The listing builds one solid part. Answer for the finished solid, in the listing's coordinates (mm). A direction names the side the tool comes from. Give positions to 0.01 mm unless a question says otherwise; leave off trailing zeros. Write each loop counter-clockwise with the first axis right and the second up, starting at its lowest first coordinate (ties: lowest second). Pieces come first, ordered by that corner, then holes. Notation, with made-up numbers: (6.25, 86.25) - (18.25, 86.25) arc R6 ccw to (18.25, 90.25) - close; hole circle Ø7 at (-28.5, 45). An arc over 180 degrees is marked (long way). Write each question's results on one line, items separated by ' | '. Start each with the question number.
Q1. Section B-B (y = 0) is taken. Determine the outline of the cut face in (x, z), plus the area to 4 significant figures.
Q2. For faces 1 (the face through (-7.215, -5.599, 6.084)), 2 (the face through (6, 6.5, 6.7)), 3 (the face through (-6, 6.5, 6.7)), determine the directions among +Z, -Z, +X, -X, +Y, -Y from which every point of the face is accessible in a straight line to the end or side of a thin tool.
Q3. Section C-C (z = 6) is taken. Determine the outline of the cut face in (x, y).
Q4. Section D-D (y = 6) is taken. Determine the outline of the cut face in (x, z), plus the area to 3 significant figures.
Q5. Flat-ended cylindrical pins translate along their axes: pin 1 Ø4 at (y, z) = (13, 5.5) entering from +X; pin 2 Ø5 at (x, z) = (4.5, 7) entering from +Y; pin 3 Ø2 at (x, y) = (-2, 9.5) entering from +Z. Find the tip coordinate at first contact, or state that the pin passes through.
Q6. Find the intervals of material crossed by probe 1 along Y at (x, z) = (0, 2.5); probe 2 along Z at (x, y) = (-4.9, 0); probe 3 along Z at (x, y) = (1.25, 9.25), in increasing order.
Q7. For a pull along Y with two mould halves and no side action, classify faces 4 (the face through (2, 4, 12)), 5 (the face through (3.926, 1.628, 5.916)), 6 (the face through (0, 8, 7)) as pulls with the +Y half, pulls with the -Y half, needs draft (parallel to the pull), parting line crosses it, or undercut.
Q8. Section A-A (x = 0) is taken. Determine the outline of the cut face in (y, z), plus the area to 3 significant figures.
Autodesk Fusion 360 part; units mm, degrees
sketch "スケッチ1" plane through (0, 0, 0) normal (0, 0, 1) x (1, 0, 0)
  line L0 (7.5, 16) -> (-7.5, 16)
  line L1 (-7.5, 16) -> (-7.5, -5.9)
  line L2 (-7.5, -5.9) -> (7.5, -5.9)
  line L3 (7.5, -5.9) -> (7.5, 16)
  line L4 (7.5, 16) -> (-7.5, -5.9) construction
  line L5 (-7.5, 16) -> (7.5, -5.9) construction
  circle A0 centre (0, 0) radius 4.25
  line L6 (-7.5, 5) -> (-4.5, 8)
  line L7 (-4.5, 8) -> (4.5, 8)
  line L8 (4.5, 8) -> (7.5, 5)
  point P0 (0, 5.05)
  dimension "d1" = 15
  dimension "d2" = 21.9
  dimension "d3" = 8.5
  dimension "d4" = 5.9
  dimension "d5" = 13.9
  dimension "d6" = 45
  dimension "d7" = 45
  dimension "d8" = 3
  dimension "d9" = 3
extrude "押し出し1" add sketch "スケッチ1" along normal blind 12 contours L1 L2 L3 L6 L7 L8
extrude "押し出し2" add sketch "スケッチ1" along normal blind 1.6 contours L0 L1 L3 L6 L7 L8
hole "穴1" at (7.5, 0, 6) direction (-1, 0, 0) diameter 2.5 depth 16 tip angle 118
fillet "フィレット1" radius 1 8 edges at (-7.5, -5.9, 6) (7.5, -5.9, 6) (7.5, 5, 6.8) (4.5, 8, 6.8) (-4.5, 8, 6.8) (-7.5, 5, 6.8) (-7.5, 16, 0.8) (7.5, 16, 0.8)
Answers below:
1) outline: (-7.5, 0) - (-4.25, 0) - (-4.25, 4.75) - (-7.5, 4.75) - close; (-7.5, 7.25) - (-4.25, 7.25) - (-4.25, 12) - (-7.5, 12) - close; (4.25, 0) - (7.5, 0) - (7.5, 4.75) - (4.25, 4.75) - close; (4.25, 7.25) - (7.5, 7.25) - (7.5, 12) - (4.25, 12) - close | area: 61.75 mm2
2) face 1: +Z, -Z, -X, -Y | face 2: +Z, +X, +Y | face 3: +Z, -X, +Y
3) outline: (-7.5, -4.9) arc R1 ccw to (-6.5, -5.9) - (6.5, -5.9) arc R1 ccw to (7.5, -4.9) - (7.5, -1.25) - (4.06, -1.25) arc R4.25 cw to (-4.06, -1.25) - (-7.5, -1.25) - close; (-7.5, 1.25) - (-4.06, 1.25) arc R4.25 cw to (4.06, 1.25) - (7.5, 1.25) - (7.5, 4.59) arc R1 ccw to (7.21, 5.29) - (4.79, 7.71) arc R1 ccw to (4.09, 8) - (-4.09, 8) arc R1 ccw to (-4.79, 7.71) - (-7.21, 5.29) arc R1 ccw to (-7.5, 4.59) - close
4) outline: (-7.5, 0) - (7.5, 0) - (7.5, 1.6) - (6.5, 1.6) - (6.5, 12) - (-6.5, 12) - (-6.5, 1.6) - (-7.5, 1.6) - close | area: 159 mm2
5) pin 1: passes through | pin 2: stops at y = 8 | pin 3: stops at z = 1.6
6) probe 1: y = -5.9 to -4.25, 4.25 to 8 | probe 2: z = 0 to 4.75, 7.25 to 12 | probe 3: z = 0 to 1.6
7) face 4: needs draft | face 5: undercut | face 6: pulls with the +Y half
8) outline: (-5.9, 0) - (-4.25, 0) - (-4.25, 12) - (-5.9, 12) - close; (4.25, 0) - (16, 0) - (16, 1.6) - (8, 1.6) - (8, 12) - (4.25, 12) - close | area: 77.6 mm2
